from build123d import *

# Parameters (mm, degrees)
SKETCH1_R           = 101.6
BOSS_EXTRUDE1_DEPTH = 12.7
CUT_EXTRUDE1_DEPTH  = 145.244271983
CIRPATTERN1_COUNT   = 6
CUT_EXTRUDE2_START  = -12.7
CUT_EXTRUDE2_DEPTH  = 12.7
CIRPATTERN2_COUNT   = 6
SKETCH4_R           = 31.75
BOSS_EXTRUDE2_DEPTH = 25.4
SKETCH7_R           = 19.05
SKETCH7_W           = 9.144
SKETCH7_H           = 5.08
CUT_EXTRUDE5_DEPTH  = 142.897378912
FILLET1_R           = 6.35


with BuildPart() as part:
    # Sketch1 → Boss-Extrude1 (new body)
    with BuildSketch(Plane(origin=(0, 0, 0), x_dir=(0, 0, -1), z_dir=(1, 0, 0))):
        Circle(SKETCH1_R)
    extrude(amount=BOSS_EXTRUDE1_DEPTH)

    # Sketch2 → Cut-Extrude1 (cut, symmetric)
    with BuildSketch(Plane(origin=(12.7, 0, 0), x_dir=(0, 0, -1), z_dir=(1, 0, 0))):
        with BuildLine():
            Line((6.35, 50.8), (6.35, 101.401368334))
            ThreePointArc((6.35, 101.401368334), (0, 101.6), (-6.35, 101.401368334))
            Line((-6.35, 101.401368334), (-6.35, 50.8))
            ThreePointArc((-6.35, 50.8), (0, 44.45), (6.35, 50.8))
        make_face()
    cut_extrude1 = extrude(amount=CUT_EXTRUDE1_DEPTH, both=True, mode=Mode.SUBTRACT)

    # CirPattern1: Cut-Extrude1 ×6 about axis
    cirpattern1_axis = Axis((12.7, 0, 0), (-1, 0, 0))
    for i in range(1, CIRPATTERN1_COUNT):
        add(cut_extrude1.rotate(cirpattern1_axis, i * 360 / CIRPATTERN1_COUNT), mode=Mode.SUBTRACT)

    # Sketch3 → Cut-Extrude2 (cut)
    with BuildSketch(Plane(origin=(12.7, 0, 0), x_dir=(0, 0, -1), z_dir=(1, 0, 0)).offset(CUT_EXTRUDE2_START)):
        with BuildLine():
            ThreePointArc((-76.2, 0), (-81.508741002, 19.399570442), (-95.955555556, 33.392983665))
            ThreePointArc((-95.955555556, 33.392983665), (-101.6, 0), (-95.955555556, -33.392983665))
            ThreePointArc((-95.955555556, -33.392983665), (-81.508741002, -19.399570442), (-76.2, 0))
        make_face()
    cut_extrude2 = extrude(amount=CUT_EXTRUDE2_DEPTH, mode=Mode.SUBTRACT)

    # CirPattern2: Cut-Extrude2 ×6 about axis
    cirpattern2_axis = Axis((0, 0, 0), (1, 0, 0))
    for i in range(1, CIRPATTERN2_COUNT):
        add(cut_extrude2.rotate(cirpattern2_axis, i * 360 / CIRPATTERN2_COUNT), mode=Mode.SUBTRACT)

    # Sketch4 → Boss-Extrude2 (add)
    with BuildSketch(Plane(origin=(12.7, 0, 0), x_dir=(0, 0, -1), z_dir=(1, 0, 0))):
        Circle(SKETCH4_R)
    extrude(amount=-BOSS_EXTRUDE2_DEPTH)

    # Sketch7 → Cut-Extrude5 (cut, through all)
    with BuildSketch(Plane.ZY.offset(12.7)):
        Circle(SKETCH7_R)
        with Locations((0, 21.033223516)):
            Rectangle(SKETCH7_W, SKETCH7_H)
    extrude(amount=-CUT_EXTRUDE5_DEPTH, mode=Mode.SUBTRACT)

    # Fillet1
    fillet1_edges = [part.edges().sort_by_distance(p)[0] for p in [
        (0, 0, 31.75),
    ]]
    fillet(fillet1_edges, radius=FILLET1_R)


solid = part.part
Read the model definition and answer for the solid it produces. Units are mm, in the model's axes. A direction names the side the tool comes from. Give positions to 0.01 mm unless a question says otherwise; leave off trailing zeros. Loops run counter-clockwise (first coordinate to the right, second up) from the corner with the lowest first, then second, coordinate; pieces in that order, holes last. Notation, with made-up numbers: (-15.75, 45) -> (43.25, 45) arc R9 ccw to (43.25, 50) -> close; hole circle Ø5 at (17.5, 1). An arc over 180 degrees is marked (long way). Use a Markdown table: item, result.
Q1. A tool of negligible diameter and unlimited length cuts with its end or side. For faces 4 (the face through (6, -76, -6.35)), 5 (the face through (6.261, -100.788, 12.819)), 6 (the face through (0, 23.573, 0)), from which of +Z, -Z, +X, -X, +Y, -Y can it reach the whole face along a straight path? Write none if from no direction.
Solved:
| item | result |
|---|---|
| face 4 | +X, -X, -Y |
| face 5 | +Z, +X, -X, -Y |
| face 6 | +X, -X |
Q2. Find the intervals of material crossed by line 1 along Z through (x, y) = (2.75, 24); line 2 along Z through (x, y) = (3.75, 0); line 3 along Y through (x, z) = (5, -70), in increasing order.
Solved:
| item | result |
|---|---|
| line 1 | z = -84.71 to -54.27, -37.8 to 37.8, 54.27 to 84.71 |
| line 2 | z = -76.2 to -19.05, 19.05 to 76.2 |
| line 3 | y = -63.12 to -47.75, -33.08 to 33.08, 47.75 to 63.12 |
Q3. Section B-B, the plane y = -78 is taken. Determine the outline of the cut face in (x, z).
Solved:
| item | result |
|---|---|
| outline | (0, -25.35) -> (12.7, -25.35) -> (12.7, -6.35) -> (0, -6.35) -> close; (0, 6.35) -> (12.7, 6.35) -> (12.7, 25.35) -> (0, 25.35) -> close |
Q4. Each of these flat-tipped pins is pushed along its axis until it touches: pin 1 (6.5 mm diameter, centred on x = 8.5, y = 78, fed in from -Z); pin 2 (4 mm diameter, centred on x = -6, z = 6.5, fed in from -Y); pin 3 (10 mm diameter, centred on x = 1, y = 23.5, fed in from +Z). Where does it stop, or does it pass through?
Solved:
| item | result |
|---|---|
| pin 1 | stops at z = -27.75 |
| pin 2 | stops at y = -31.63 |
| pin 3 | stops at z = 89.01 |
Q5. Section D-D, the plane z = -53 is taken. Determine the outline of the cut face in (x, y).
Solved:
| item | result |
|---|---|
| outline | (0, -61.11) -> (12.7, -61.11) -> (12.7, -37.93) -> (0, -37.93) -> close; (0, -23.27) -> (12.7, -23.27) -> (12.7, 23.27) -> (0, 23.27) -> close; (0, 37.93) -> (12.7, 37.93) -> (12.7, 61.11) -> (0, 61.11) -> close |
Q6. Section A-A, the plane z = 0 is taken. Determine the outline of the cut face in (x, y), then the cut area to 3 significant figures.
Solved:
| item | result |
|---|---|
| outline | (-12.7, -31.75) -> (-6.35, -31.75) arc R6.35 cw to (0, -38.1) -> (0, -44.45) -> (12.7, -44.45) -> (12.7, -19.05) -> (-12.7, -19.05) -> close; (-12.7, 23.57) -> (12.7, 23.57) -> (12.7, 44.45) -> (0, 44.45) -> (0, 38.1) arc R6.35 cw to (-6.35, 31.75) -> (-12.7, 31.75) -> close |
| area | 870 mm^2 |
Q7. Determine the mould class of faces 1 (the face through (-9.481, -30.995, 6.883)), 2 (the face through (6.26, -100.81, -12.64)), 3 (the face through (0, 21, 4.572)) for opening direction Z: pulls with the +Z half, pulls with the -Z half, needs draft (parallel to the pull), parting line crosses it, or undercut.
Solved:
| item | result |
|---|---|
| face 1 | parting line crosses it |
| face 2 | pulls with the -Z half |
| face 3 | undercut |
Q8. Section C-C, the plane x = -9 is taken. Determine the outline of the cut face in (y, z), then the cut area to 3 significant figures.
Solved:
| item | result |
|---|---|
| outline | circle Ø63.5 at (0, 0); hole (18.49, -4.57) -> (23.57, -4.57) -> (23.57, 4.57) -> (18.49, 4.57) arc R19.05 ccw (long way) to start |
| area | 1,980 mm^2 |
